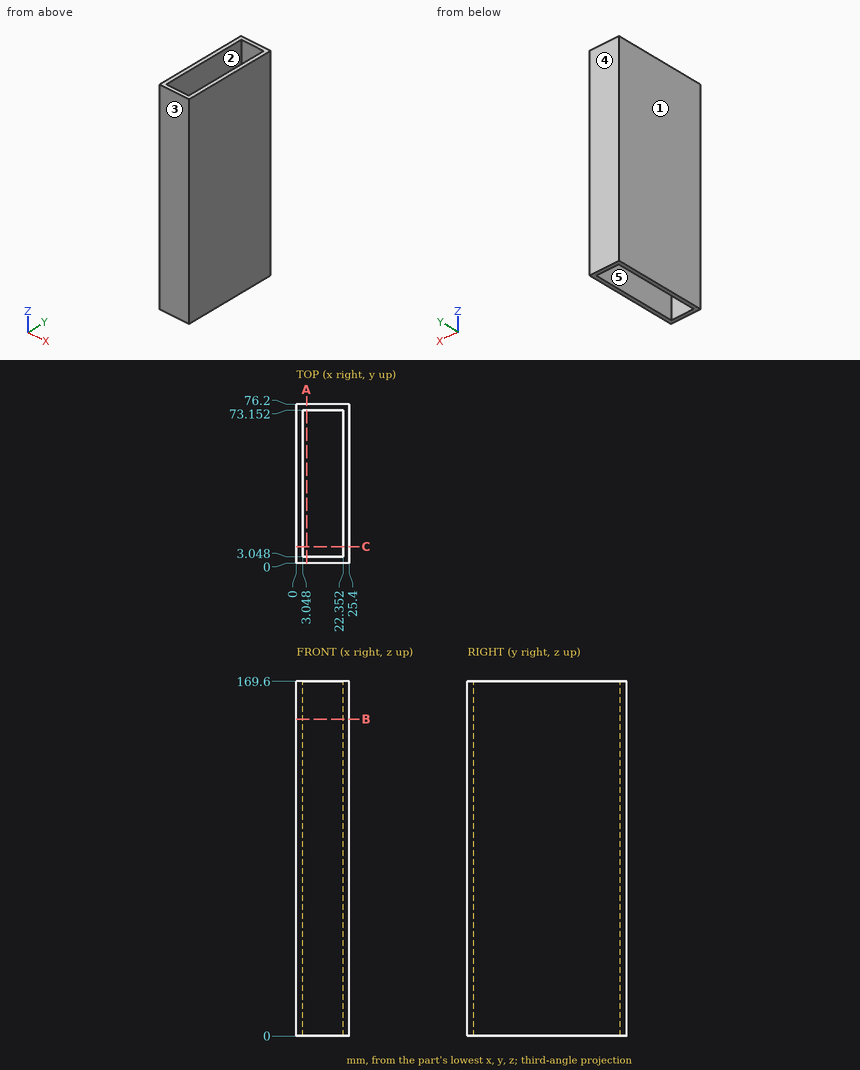
Geometry: see drawing. Coordinates: mm, zero at the bounding-box minimum. A direction names the side the tool comes from. Round coordinates to 2 decimals unless told otherwise and drop trailing zeros. Order: outer loops, then holes, each group sorted by start corner. A loop starts at its lowest first (then second) coordinate and runs counter-clockwise, first axis right, second up. Notation, with made-up numbers: (0, -31) -> (54, -31) arc R25 ccw to (54, -14) -> close; hole circle Ø2 at (65.25, -33). An arc over 180 degrees is marked (long way). Write each question's results on one line, items separated by ' | '.
Q1. Ray query, line 1 along X through (y, z) = (31.5, 71.5); line 2 along Y through (x, z) = (7, 161). Return the intervals inside material, ascending.
Response values:
line 1: 0 to 3.05, 22.35 to 25.4 | line 2: 0 to 3.05, 73.15 to 76.2
Q2. Pull-direction query (Y, two-part tool) for the marked faces 1, 2 and 3; classes: released by +Y, released by -Y, zero draft, split by the parting line, or undercut.
Response values:
face 1: zero draft | face 2: undercut | face 3: released by -Y
Q3. Section query B-B (z = 151.5). Output: boundary loops of the cut face in (x, y), and give its area (3 significant figures).
Response values:
outline: (0, 0) -> (25.4, 0) -> (25.4, 76.2) -> (0, 76.2) -> close; hole (3.05, 3.05) -> (22.35, 3.05) -> (22.35, 73.15) -> (3.05, 73.15) -> close | area: 582 mm²
Q4. Pin query (flat end, axial travel): pin 1 Ø1 at (x, z) = (10, 118.5) entering from -Y. Return the tip coordinate at first contact, or that it passes through.
Response values:
pin 1: y = 0
Q5. Section query C-C (y = 8). Output: boundary loops of the cut face in (x, z).
Response values:
outline: (0, 0) -> (3.05, 0) -> (3.05, 169.6) -> (0, 169.6) -> close; (22.35, 0) -> (25.4, 0) -> (25.4, 169.6) -> (22.35, 169.6) -> close
Q6. Access query for the marked faces 4 and 5. Directions: +Z, -Z, +X, -X, +Y, -Y. A direction counts if a zero-diameter tool reaches every point of the face in a straight line with its end or side. Return the directions, or none.
Response values:
face 4: +Z, -Z, +X, -X, +Y | face 5: +Z, -Z
Q7. Section query A-A (x = 5). Output: boundary loops of the cut face in (y, z).
Response values:
outline: (0, 0) -> (3.05, 0) -> (3.05, 169.6) -> (0, 169.6) -> close; (73.15, 0) -> (76.2, 0) -> (76.2, 169.6) -> (73.15, 169.6) -> close
